Geometry check sheet. Reference: the model listing, model coordinates, mm. A direction names the side the tool comes from. Round coordinates to 2 decimals unless told otherwise and drop trailing zeros. Write each loop counter-clockwise with the first axis right and the second up, starting at its lowest first coordinate (ties: lowest second). Pieces come first, ordered by that corner, then holes. Notation, with made-up numbers: (25, -27) - (63, -27) arc R5 ccw to (63, -22) - close; hole circle Ø2 at (-33.5, 67.25). An arc over 180 degrees is marked (long way). Return JSON: item names as keys, results as strings.
Autodesk Inventor part; units mm, degrees
ref_plane "Work Plane1" through (0, 0, -15) normal (0, 0, 1) x (1, 0, 0)
ref_plane "YZ Plane" through (0, 0, 0) normal (1, 0, 0) x (0, 1, 0)
ref_plane "XZ Plane" through (0, 0, 0) normal (0, 1, 0) x (-1, 0, 0)
sketch "Sketch1" plane through (0, 0, 0) normal (0, 0, 1) x (1, 0, 0)
  line L0 (0, 0) -> (25, 0)
  line L1 (25, 0) -> (25, 40)
  line L2 (25, 40) -> (0, 40)
  line L3 (0, 40) -> (0, 0)
  dimension "d1" = 25
  dimension "d2" = 40
  dimension "d3" = 25
extrude "Extrusion1" add sketch "Sketch1" against normal blind 30
sketch "Sketch2" plane through (25, 0, 0) normal (1, 0, 0) x (0, 0, -1)
  line L0 (0, 0) -> (30, 0)
  circle A0 centre (15, 6.56) radius 2.46
extrude "Extrusion2" cut sketch "Sketch2" against normal blind 30
sketch "Sketch3" plane through (0, 0, 0) normal (-1, 0, 0) x (0, 0, 1)
  line L0 (0, 0) -> (-30, 0)
  line L1 (-25.05, 0) -> (-4.95, 0)
  line L2 (-4.95, 0) -> (-4.95, 33.12)
  line L3 (-4.95, 33.12) -> (-25.05, 33.12)
  line L4 (-25.05, 33.12) -> (-25.05, 0)
  dimension "d11" = 20.1
extrude "Extrusion3" cut sketch "Sketch3" against normal blind 20
sketch "Sketch4" plane through (0, 0, 0) normal (0, -1, 0) x (1, 0, 0)
  line L0 (20, -4.95) -> (20, -25.05)
  line L1 (20, -15) -> (25, -15)
  line L2 (25, 0) -> (25, -30)
  line L3 (20, -8.025) -> (25, -8.025)
  line L4 (25, -8.025) -> (25, -21.975)
  line L5 (25, -21.975) -> (20, -21.975)
  line L6 (20, -21.975) -> (20, -8.025)
  line L7 (20, -8.025) -> (25, -21.975) construction
  line L8 (25, -8.025) -> (20, -21.975) construction
  line L9 (25, -12.54) -> (25, -17.46)
  point P0 (0, 0)
  point P1 (22.5, -15)
  dimension "d14" = 13.95
extrude "Extrusion4" add sketch "Sketch4" along normal blind 15
sketch "Sketch5" plane through (20, 0, 0) normal (-1, 0, 0) x (0, 0, 1)
  circle A0 centre (-15, 6.56) radius 2.46
  circle A1 centre (-15, 6.56) radius 4.7025
  circle A2 centre (-15, 6.56) radius 2.46
  circle A3 centre (-15, 6.56) radius 2.46
  point P0 (0, 0)
  dimension "d17" = 9.405
extrude "Extrusion5" cut sketch "Sketch5" against normal blind 2.1
sketch "Sketch6" plane through (25, 0, 0) normal (1, 0, 0) x (0, 0, -1)
  circle A0 centre (15, 6.56) radius 4.7025
  line L0 (15, 6.56) -> (15, 23.56)
  circle A1 centre (15, 23.56) radius 2.46
  point P0 (0, 0)
  dimension "d20" = 17
  dimension "d21" = 4.92
extrude "Extrusion6" cut sketch "Sketch6" against normal blind 10 contours A1
sketch "Sketch7" plane through (20, 0, 0) normal (-1, 0, 0) x (0, 0, 1)
  circle A0 centre (-15, 23.56) radius 2.46
  circle A1 centre (-15, 23.56) radius 4.7025
  point P0 (0, 0)
  dimension "d24" = 9.405
extrude "Extrusion7" cut sketch "Sketch7" against normal blind 2.1
sketch "Sketch9" plane through (25, 0, 0) normal (1, 0, 0) x (0, 0, -1)
  circle A0 centre (15, 6.56) radius 2.46
  circle A1 centre (15, 6.56) radius 2.46
  circle A2 centre (15, 23.56) radius 2.46
  circle A3 centre (15, 23.56) radius 2.46
  line L0 (30, 40) -> (30, 0)
  line L1 (30, 0) -> (30, 40)
  line L2 (30, 40) -> (0, 40)
  line L3 (0, 40) -> (0, 0)
  line L4 (0, 0) -> (8.025, 0)
  line L5 (21.975, 0) -> (21.975, -15)
  line L6 (21.975, -15) -> (8.025, -15)
  line L7 (8.025, -15) -> (8.025, 0)
  line L8 (0, 0) -> (8.025, 0)
  line L9 (21.975, 0) -> (30, 0)
extrude "Extrusion8" add sketch "Sketch9" along normal blind 5
sketch "Sketch10" plane through (0, 40, 0) normal (0, 1, 0) x (1, 0, 0)
  line L0 (0, 30) -> (30, 30)
  line L1 (30, 0) -> (0, 0)
  line L2 (0, 30) -> (30, 30)
  line L3 (30, 30) -> (30, 0)
  line L4 (30, 0) -> (0, 0)
  line L5 (0, 0) -> (0, 30)
extrude "Extrusion9" add sketch "Sketch10" along normal blind 30
sketch "Sketch12" plane through (30, 0, 0) normal (1, 0, 0) x (0, 0, -1)
  circle A0 centre (15, 6.56) radius 2.46
  line L0 (15, 6.56) -> (15, 15.06)
  circle A1 centre (15, 15.06) radius 2.525
  point P0 (0, 0)
  dimension "d31" = 8.5
  dimension "d33" = 5.05
extrude "Extrusion10" cut sketch "Sketch12" against normal blind 30 contours A1
sketch "Sketch15" plane through (0, 0, -25.05) normal (-1, 0, 0) x (0, 0, 1)
  line L0 (0, 33.12) -> (20.1, 33.12)
  line L1 (20.1, 33.12) -> (20.1, 0)
  line L2 (0, 33.12) -> (20.1, 33.12)
  line L3 (20.1, 33.12) -> (20.1, 31.1)
  line L4 (20.1, 31.1) -> (0, 31.1)
  line L5 (0, 31.1) -> (0, 33.12)
  point P0 (25.05, 0)
  dimension "d57" = 2.02
extrude "Extrusion13" add sketch "Sketch15" against normal blind 20
sketch "Sketch17" plane through (0, 0, 0) normal (0, 0, 1) x (1, 0, 0)
  line L0 (0, 70) -> (30, 70)
  line L1 (30, 70) -> (50.0622, 90.0622)
  line L2 (30, 70) -> (80, 70) construction
  line L3 (11.9522, 97.2454) -> (0, 85.2932)
  line L4 (0, 70) -> (0, 85.2932)
  line L5 (0, 70) -> (0, 0)
  line L6 (0, 70) -> (30, 70)
  line L7 (10.923, 112.2849) -> (0, 120.567)
  line L8 (50.0622, 105.3553) -> (50.0622, 120.567)
  line L9 (50.0622, 105.3553) -> (50.0622, 90.0622)
  arc A0 (11.9522, 97.2454) -> (10.923, 112.2849) centre (4.8811, 104.3165) ccw
  line L10 (0, 174.567) -> (30, 174.567)
  line L11 (30, 174.567) -> (50.0622, 120.567)
  line L12 (6, 171.567) -> (0, 174.567)
  line L13 (6, 123.567) -> (0, 120.567)
  line L14 (6, 123.567) -> (12, 147.567)
  line L15 (6, 171.567) -> (12, 147.567)
  dimension "d61" = 45
  dimension "d62" = 32.0271
  dimension "d72" = 10
extrude "Extrusion14" add sketch "Sketch17" against normal blind 30
sketch "Sketch24" plane through (0, 0, 0) normal (0, 0, 1) x (1, 0, 0)
  line L0 (30, 70) -> (50.0622, 90.0622)
  line L1 (30, 70) -> (50.0622, 90.0622)
  line L2 (50.0622, 90.0622) -> (50.0622, 120.567)
  line L3 (50.0622, 90.0622) -> (50.0622, 120.567)
  line L4 (30, 174.567) -> (50.0622, 120.567)
  line L5 (50.0622, 120.567) -> (30, 174.567)
  line L6 (30, 174.567) -> (0, 174.567)
  line L7 (30, 174.567) -> (0, 174.567)
  line L8 (0, 174.567) -> (6, 171.567)
  line L9 (0, 174.567) -> (6, 171.567)
  line L10 (12, 147.567) -> (6, 171.567)
  line L11 (6, 171.567) -> (12, 147.567)
  line L12 (12, 147.567) -> (6, 123.567)
  line L13 (12, 147.567) -> (6, 123.567)
  line L14 (6, 123.567) -> (0, 120.567)
  line L15 (6, 123.567) -> (0, 120.567)
  line L16 (0, 120.567) -> (10.923, 112.2849)
  line L17 (0, 120.567) -> (10.923, 112.2849)
  line L18 (0, 85.2932) -> (11.9522, 97.2454)
  line L19 (11.9522, 97.2454) -> (0, 85.2932)
  line L20 (0, 85.2932) -> (0, 55.2932)
  line L21 (0, 0) -> (0, 85.2932)
  line L22 (0, 55.2932) -> (30, 55.2932)
  line L23 (30, 0) -> (30, 70)
  line L24 (30, 55.2932) -> (30, 70)
  arc A0 (11.9522, 97.2454) -> (10.923, 112.2849) centre (4.8811, 104.3165) ccw
  dimension "d106" = 30
extrude "Extrusion15" add sketch "Sketch24" along normal blind 30
ref_plane "Work Plane1" through (0, 0, -15) normal (0, 0, 1) x (1, 0, 0)
mirror "Mirror1" about plane through (0, 0, -15) normal (0, 0, 1) of "Extrusion15"
properties part number "rec_c_48mm_x_90mm"
(1) Release check for a two-part mould opening along Y. For faces 6 (the face through (10, 15, -4.95)), 7 (the face through (15, 55.293, 15)), 8 (the face through (25.07, 15.171, -12.477)) record: pulls with the +Y half, pulls with the -Y half, needs draft (parallel to the pull), parting line crosses it, or undercut.
Response values:
{"face 6": "needs draft", "face 7": "pulls with the -Y half", "face 8": "undercut"}
(2) Section check C-C, the plane z = -52. Enter the section's corners in (x, y), plus the area to 3 significant figures.
Response values:
{"outline": "(0, 55.29) - (30, 55.29) - (30, 70) - (50.06, 90.06) - (50.06, 120.57) - (30, 174.57) - (0, 174.57) - (6, 171.57) - (12, 147.57) - (6, 123.57) - (0, 120.57) - (10.92, 112.28) arc R10 cw to (11.95, 97.25) - (0, 85.29) - close", "area": "4,160 mm^2"}
(3) Section check D-D, the plane z = -15. Give the number of separate pieces and of enclosed holes in the cut face, plus the area to 3 significant figures.
Response values:
{"separate pieces": "4", "enclosed holes": "0", "area": "5,180 mm^2"}
(4) Material ranges on line 1 along Y through (x, z) = (27, -15) (3 decimals); line 2 along Z through (x, y) = (27, 23.56); line 3 along Z through (x, y) = (13.5, 19.5), recorded low to high. Write a range as [from, to].
Response values:
{"line 1": "y = [-15, 4.1], [9.02, 12.535], [17.585, 21.1], [26.02, 174.567]", "line 2": "z = [-30, -17.46], [-12.54, 0]", "line 3": "z = [-30, -25.05], [-4.95, 0]"}
(5) Access from +Z, -Z, +X, -X, +Y, -Y to the whole of each face (thin tool, end or side, straight path). Record for faces 1 (the face through (8.96, 135.4, -14.37)), 2 (the face through (10, 16, -25.05)), 3 (the face through (15, 55.293, -45)), 4 (the face through (22.1, 21.5, -13)), 5 (the face through (25, -8, -8.025)).
Response values:
{"face 1": "+Z, -Z, -X", "face 2": "-X, -Y", "face 3": "-Z, +X, -X, -Y", "face 4": "-X", "face 5": "+Z, +X, -X, -Y"}
(6) Gauge pin test, flat ends, axial feed: pin 1 (6.5 mm diameter, centred on x = 19, z = -26, fed in from -Y); pin 2 (9 mm diameter, centred on x = 14.5, y = 14, fed in from +Z); pin 3 (9 mm diameter, centred on x = 14.5, z = 11, fed in from -Y); pin 4 (10 mm diameter, centred on y = 71.5, z = -15.5, fed in from -X). Record the tip position at first contact, or that the pin passes through.
Response values:
{"pin 1": "stops at y = 0", "pin 2": "stops at z = 0", "pin 3": "stops at y = 55.29", "pin 4": "stops at x = 0"}
(7) Section check B-B, the plane y = 15.06. Enter the section's corners in (x, z) (3 decimals), plus the area to 4 significant figures.
Response values:
{"outline": "(0, -30) - (30, -30) - (30, -17.525) - (20, -17.525) - (20, -25.05) - (0, -25.05) - close; (0, -4.95) - (20, -4.95) - (20, -12.475) - (30, -12.475) - (30, 0) - (0, 0) - close", "area": "447.5 mm^2"}
(8) Section check A-A, the plane x = 26.5. Enter the section's corners in (y, z) (3 decimals), plus the area to 3 significant figures.
Response values:
{"outline": "(-15, -21.975) - (0, -21.975) - (0, -30) - (55.293, -30) - (55.293, -60) - (174.567, -60) - (174.567, 30) - (55.293, 30) - (55.293, 0) - (0, 0) - (0, -8.025) - (-15, -8.025) - close; hole circle Ø4.92 at (6.56, -15); hole circle Ø5.05 at (15.06, -15); hole circle Ø4.92 at (23.56, -15)", "area": "12,500 mm^2"}
